Build history of the part. All positions in model axes, mm. A direction names the side the tool comes from. Coordinates: 2 decimals unless noted, no trailing zeros. Loops run counter-clockwise (first coordinate to the right, second up) from the corner with the lowest first, then second, coordinate; pieces in that order, holes last. Notation, with made-up numbers: (-19, 75.5) - (-10, 75.5) arc R37 ccw to (-10, 114.5) - close; hole circle Ø8 at (55, 49.5). An arc over 180 degrees is marked (long way). One line per item, written item: value.
Autodesk Inventor part; units mm, degrees
ref_plane "YZ Plane" through (0, 0, 0) normal (1, 0, 0) x (0, 1, 0)
ref_plane "XZ Plane" through (0, 0, 0) normal (0, 1, 0) x (-1, 0, 0)
ref_plane "XY Plane" through (0, 0, 0) normal (0, 0, 1) x (1, 0, 0)
sketch "Sketch1" plane through (0, 0, 0) normal (0, 0, 1) x (1, 0, 0)
  line L0 (0, 0) -> (-114.3, 0)
  line L1 (-114.3, 0) -> (-114.3, 114.3)
  line L2 (-114.3, 114.3) -> (0, 114.3)
  line L3 (0, 114.3) -> (0, 0)
  line L4 (-3.81, 3.81) -> (-110.49, 3.81)
  line L5 (-110.49, 3.81) -> (-110.49, 110.49)
  line L6 (-110.49, 110.49) -> (-3.81, 110.49)
  line L7 (-3.81, 110.49) -> (-3.81, 3.81)
  dimension "d0" = 3.81
  dimension "d1" = 3.81
  dimension "d2" = 3.81
  dimension "d3" = 3.81
  dimension "d4" = 114.3
  dimension "d5" = 114.3
extrude "Extrusion1" add sketch "Sketch1" along normal blind 3.81 contours L0 L1 L2 L3 | L4 L5 L6 L7
sketch "Sketch2" plane through (0, 0, 3.81) normal (0, 0, 1) x (1, 0, 0)
  line L0 (-4.064, 4.064) -> (-110.236, 4.064)
  line L1 (-110.236, 4.064) -> (-110.236, 110.236)
  line L2 (-110.236, 110.236) -> (-4.064, 110.236)
  line L3 (-4.064, 110.236) -> (-4.064, 4.064)
  line L4 (-114.3, 114.3) -> (-114.3, 0)
  line L5 (0, 114.3) -> (-114.3, 114.3)
  line L6 (0, 0) -> (0, 114.3)
  line L7 (-114.3, 0) -> (0, 0)
  dimension "d8" = 4.064
  dimension "d9" = 4.064
  dimension "d10" = 4.064
  dimension "d11" = 4.064
extrude "Extrusion2" add sketch "Sketch2" along normal blind 3.81 contours L0 L1 L2 L3
fillet "Fillet1" radius 3.175 4 edges at (-4.064, 110.236, 5.715) (-110.236, 110.236, 5.715) (-110.236, 4.064, 5.715) (-4.064, 4.064, 5.715)
sketch "Sketch3" plane through (0, 0, 0) normal (0, 0, -1) x (-1, 0, 0)
  circle A0 centre (109.22, 85.725) radius 1.651
  circle A1 centre (109.22, 28.575) radius 1.651
  line L0 (114.3, 0) -> (114.3, 114.3)
  line L1 (114.3, 114.3) -> (0, 114.3)
  circle A2 centre (5.08, 85.725) radius 1.651
  circle A3 centre (5.08, 28.575) radius 1.651
  line L2 (0, 114.3) -> (0, 0)
  line L3 (0, 0) -> (114.3, 0)
  dimension "d15" = 3.302
  dimension "d16" = 57.15
  dimension "d17" = 57.15
  dimension "d18" = 104.14
  dimension "d19" = 104.14
  dimension "d20" = 28.575
  dimension "d21" = 114.3
  dimension "d22" = 5.08
  dimension "d23" = 5.08
  dimension "d24" = 5.08
  dimension "d37" = 114.3
  dimension "d38" = 114.3
  dimension "d39" = 114.3
  dimension "d40" = 114.3
extrude "Extrusion3" cut sketch "Sketch3" against normal up to surface (7.62 mm away) contours A0 | A1 | A2 | A3
fillet "Fillet2" radius 3.175 8 edges at (-4.064, 27.2736, 5.715) (-4.064, 29.8764, 5.715) (-4.064, 84.4236, 5.715) (-4.064, 87.0264, 5.715) (-110.236, 87.0264, 5.715) (-110.236, 84.4236, 5.715) (-110.236, 29.8764, 5.715) (-110.236, 27.2736, 5.715)
equation "\"d1\" = d0"
equation "\"d2\" = d0"
equation "\"d3\" = d0"
equation "\"d16\" = d17"
equation "\"d19\" = d18"
equation "\"d23\" = d22"
equation "\"d24\" = d22"
properties part number "Lid"
Item 1: Probe probe 1 along Y at (x, z) = (-109.22, 3.75); probe 2 along Y at (x, z) = (-109.22, 4); probe 3 along Y at (x, z) = (-65.5, 4.5). List the from-to ranges inside material, lowest first. Write a range as from..to.
Check result:
probe 1: y = 0..26.92, 30.23..84.07, 87.38..114.3
probe 2: y = 4.91..26.59, 30.56..83.74, 87.71..109.39
probe 3: y = 4.06..110.24
Item 2: Tool access for faces 1 (the face through (-109.75, 88.35, 5.69)), 2 (the face through (-110.236, 57, 6)), 3 (the face through (-4.064, 99, 6)), 4 (the face through (-5.02, 4.97, 5.74)): list every direction of +Z, -Z, +X, -X, +Y, -Y with a clear straight run to the whole face (end or side of a thin tool).
Check result:
face 1: +Z, -X
face 2: +Z, -X, +Y, -Y
face 3: +Z, +X, +Y, -Y
face 4: +Z, +X, -Y
Item 3: Pull direction Y, two halves, no side cores. Call faces 5 (the face through (-110.236, 16, 6)), 6 (the face through (-109.775, 83.057, 5.688)), 7 (the face through (-58, 110.236, 6)): released by +Y, released by -Y, zero draft, split by the parting line, or undercut.
Check result:
face 5: zero draft
face 6: undercut
face 7: released by +Y
Item 4: Cut at B-B, the plane z = 5.75. Write the cut outline in (x, y) (3 decimals).
Check result:
outline: (-110.236, 7.239) arc R3.175 ccw to (-107.061, 4.064) - (-7.239, 4.064) arc R3.175 ccw to (-4.064, 7.239) - (-4.064, 24.259) arc R3.175 ccw to (-5.819, 27.098) arc R1.651 cw to (-5.819, 30.052) arc R3.175 ccw to (-4.064, 32.891) - (-4.064, 81.409) arc R3.175 ccw to (-5.819, 84.248) arc R1.651 cw to (-5.819, 87.202) arc R3.175 ccw to (-4.064, 90.041) - (-4.064, 107.061) arc R3.175 ccw to (-7.239, 110.236) - (-107.061, 110.236) arc R3.175 ccw to (-110.236, 107.061) - (-110.236, 90.041) arc R3.175 ccw to (-108.481, 87.202) arc R1.651 cw to (-108.481, 84.248) arc R3.175 ccw to (-110.236, 81.409) - (-110.236, 32.891) arc R3.175 ccw to (-108.481, 30.052) arc R1.651 cw to (-108.481, 27.098) arc R3.175 ccw to (-110.236, 24.259) - close
Item 5: Drop flat-ended pins along their axis: P1, Ø4, axis at x = -46.5, z = 6, coming from the -Y side; P2, Ø1.9, axis at y = 18.5, z = 6.5, coming from the -X side; P3, Ø1.9, axis at y = 96, z = 6, coming from the +X side. Give the stop position or say it passes through.
Check result:
P1: stops at y = 4.06
P2: stops at x = -110.24
P3: stops at x = -4.06
Item 6: Cut at A-A, the plane x = -95. Write the cut outline in (y, z), then the cut area to 3 significant figures.
Check result:
outline: (0, 0) - (114.3, 0) - (114.3, 3.81) - (110.24, 3.81) - (110.24, 7.62) - (4.06, 7.62) - (4.06, 3.81) - (0, 3.81) - close
area: 840 mm^2
Item 7: Cut at C-C, the plane y = 34.5. Write the cut outline in (x, z), then the cut area to 3 significant figures.
Check result:
outline: (-114.3, 0) - (0, 0) - (0, 3.81) - (-4.06, 3.81) - (-4.06, 7.62) - (-110.24, 7.62) - (-110.24, 3.81) - (-114.3, 3.81) - close
area: 840 mm^2
